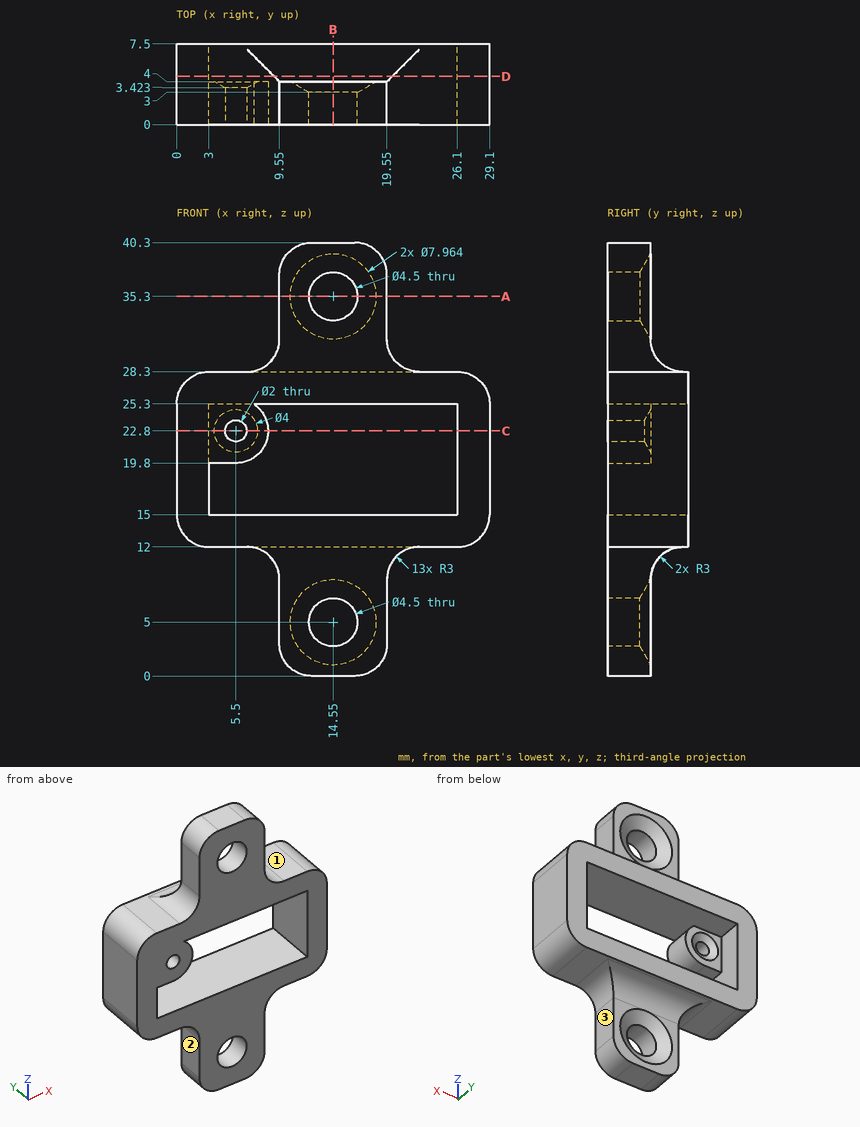
Part print with two shaded views. Sizes in mm from the minimum x, y, z corner. A direction names the side the tool comes from. Coordinates: 2 decimals unless noted, no trailing zeros. Order: outer loops, then holes, each group sorted by start corner. A loop starts at its lowest first (then second) coordinate and runs counter-clockwise, first axis right, second up. Notation, with made-up numbers: (40.5, -28.5) - (98.5, -28.5) arc R20 cw to (98.5, -23.5) - close; hole circle Ø8 at (17.25, 74). An arc over 180 degrees is marked (long way). Write item = value, one per line. Start each with the question number.
1) Saw through at A-A on z = 35.3. Write the cut outline in (x, y).
2) Saw through at B-B on x = 14.55. Count the separate pieces of the cut face and the enclosed holes in it, then the cut area to 3 significant figures.
3) Saw through at C-C on z = 22.8. Write the cut outline in (x, y).
4) Saw through at D-D on y = 4.5. Write the cut outline in (x, z), then the cut area to 3 significant figures.
5) Wall check: line 1 along X through (y, z) = (1, 22.8); line 2 along X through (y, z) = (6.5, 24); line 3 along X through (y, z) = (1.9, 5). Give the ranges that are in metal, low to high. Write a range as from..to.
6) Flat gauge pins, fed straight in: pin 1 Ø4.5 at (y, z) = (1.5, 6) entering from -X; pin 2 Ø4.5 at (y, z) = (2, 5) entering from +X; pin 3 Ø1 at (y, z) = (3.5, 28) entering from +X. Where does each tip first touch, or does it go through?
7) 3-axis set-ups, long thin cutter, end or side, ignore diameter. For the marked faces 1, 2 and 3: which of +Z, -Z, +X, -X, +Y, -Y reach the whole face in a straight line?
From the geometry:
q1.outline = (9.55, 0) - (12.3, 0) - (12.3, 3) - (10.57, 4) - (9.55, 4) - close; (16.8, 0) - (19.55, 0) - (19.55, 4) - (18.53, 4) - (16.8, 3) - close
q2.separate_pieces = 4
q2.enclosed_holes = 0
q2.area = 105 mm^2
q3.outline = (0, 0) - (4.5, 0) - (4.5, 3.42) - (3.5, 4) - (3, 4) - (3, 7.5) - (0, 7.5) - close; (6.5, 0) - (8.5, 0) - (8.5, 4) - (7.5, 4) - (6.5, 3.42) - close; (26.1, 0) - (29.1, 0) - (29.1, 7.5) - (26.1, 7.5) - close
q4.outline = (0, 15) arc R3 ccw to (3, 12) - (6.55, 12) arc R3 cw to (9.05, 10.66) - (20.05, 10.66) arc R3 cw to (22.55, 12) - (26.1, 12) arc R3 ccw to (29.1, 15) - (29.1, 25.3) arc R3 ccw to (26.1, 28.3) - (22.55, 28.3) arc R3 cw to (20.05, 29.64) - (9.05, 29.64) arc R3 cw to (6.55, 28.3) - (3, 28.3) arc R3 ccw to (0, 25.3) - close; hole (3, 15) - (26.1, 15) - (26.1, 25.3) - (3, 25.3) - close
q4.area = 262 mm^2
q5.line_1 = 0..4.5, 6.5..8.5, 26.1..29.1
q5.line_2 = 0..3, 26.1..29.1
q5.line_3 = 9.55..12.3, 16.8..19.55
q6.pin_1 = 9.55
q6.pin_2 = 19.55
q6.pin_3 = 28.14
q7.face_1 = +Z, +Y
q7.face_2 = -Z, -X, +Y, -Y
q7.face_3 = -Z, +X, +Y, -Y
